```python
from build123d import *

# Parameters (mm, degrees)
SKETCH2_W             = 90
SKETCH2_H             = 23
BOSS_EXTRUDE2_DEPTH   = 5
SKETCH4_W             = 90
SKETCH4_H             = 5
BOSS_EXTRUDE3_DEPTH   = 35
M8X1_0_TAPPED_HOLE1_D = 7
M8X1_0_TAPPED_HOLE2_D = 7


with BuildPart() as part:
    # Sketch2 → Boss-Extrude2 (new body)
    with BuildSketch(Plane.XY):
        with Locations((0, -11.5)):
            Rectangle(SKETCH2_W, SKETCH2_H)
    extrude(amount=BOSS_EXTRUDE2_DEPTH)

    # Sketch4 → Boss-Extrude3 (add)
    with BuildSketch(Plane.XY.offset(5)):
        with Locations((0, -20.5)):
            Rectangle(SKETCH4_W, SKETCH4_H)
    extrude(amount=BOSS_EXTRUDE3_DEPTH)

    # M8x1.0 Tapped Hole1 (through all)
    with Locations(Plane.XY.offset(5)):
        with Locations((-25, -8), (25, -8)):
            Hole(M8X1_0_TAPPED_HOLE1_D / 2)

    # M8x1.0 Tapped Hole2 (through all)
    with Locations(Plane(origin=(0, -18, 0), x_dir=(1, 0, 0), z_dir=(0, 1, 0))):
        with Locations((-25, -25), (25, -25)):
            Hole(M8X1_0_TAPPED_HOLE2_D / 2)


solid = part.part
```
Source: CAD feature listing. Evaluate the final solid. Frame: model axes, mm. A direction names the side the tool comes from. Coordinates: 2 decimals unless noted, no trailing zeros. Write each loop counter-clockwise with the first axis right and the second up, starting at its lowest first coordinate (ties: lowest second). Pieces come first, ordered by that corner, then holes. Notation, with made-up numbers: (56, 54) - (66, 54) arc R6 cw to (66, 60) - close; hole circle Ø8 at (-16, 50). An arc over 180 degrees is marked (long way). Answer as a JSON object with one key per item and string values.
Q1. First-contact query: pin 1 Ø2 at (x, y) = (16.5, -9.5) entering from -Z; pin 2 Ø9 at (x, y) = (-9, -5.5) entering from +Z; pin 3 Ø10.5 at (x, z) = (-12.5, 27) entering from +Y. Flat tips, straight axial feed; report the tip coordinate or a pass-through.
Ans:
{"pin 1": "stops at z = 0", "pin 2": "stops at z = 5", "pin 3": "stops at y = -18"}
Q2. Material intervals for line 1 (X direction, y = -21.5, z = 25); line 2 (Y direction, x = -25, z = 3); line 3 (Z direction, x = -25, y = -20.75), sorted ascending. Write a range as [from, to].
Ans:
{"line 1": "x = [-45, -28.5], [-21.5, 21.5], [28.5, 45]", "line 2": "y = [-23, -11.5], [-4.5, 0]", "line 3": "z = [0, 21.5], [28.5, 40]"}
Q3. Section query D-D, the plane z = 20. Output: boundary loops of the cut face in (x, y).
Ans:
{"outline": "(-45, -23) - (45, -23) - (45, -18) - (-45, -18) - close"}
Q4. Section query B-B, the plane z = 25. Output: boundary loops of the cut face in (x, y).
Ans:
{"outline": "(-45, -23) - (-28.5, -23) - (-28.5, -18) - (-45, -18) - close; (-21.5, -23) - (21.5, -23) - (21.5, -18) - (-21.5, -18) - close; (28.5, -23) - (45, -23) - (45, -18) - (28.5, -18) - close"}
Q5. Draft query along Z for faces 1 (the flat face through (-1, -18, 22)), 2 (the flat face through (-1, -11, 0)), 3 (the cylindrical face through (23.12, -20.53, 22.05)). Return one class per face: released by +Z, released by -Z, zero draft, split by the parting line, or undercut.
Ans:
{"face 1": "zero draft", "face 2": "released by -Z", "face 3": "undercut"}
Q6. Set-up query: faces 4 (the flat face through (-1, -23, 20)), 5 (the flat face through (-1, -9, 5)). Return all of +Z, -Z, +X, -X, +Y, -Y with unobstructed straight access to the full face (end or side cutting, diameter ignored); none if empty.
Ans:
{"face 4": "+Z, -Z, +X, -X, -Y", "face 5": "+Z, +X, -X, +Y"}
Q7. Section query C-C, the plane y = -8. Output: boundary loops of the cut face in (x, z), plus the area to 3 significant figures.
Ans:
{"outline": "(-45, 0) - (-28.5, 0) - (-28.5, 5) - (-45, 5) - close; (-21.5, 0) - (21.5, 0) - (21.5, 5) - (-21.5, 5) - close; (28.5, 0) - (45, 0) - (45, 5) - (28.5, 5) - close", "area": "380 mm2"}
Q8. Section query A-A, the plane x = -25. Output: boundary loops of the cut face in (y, z), plus the area to 3 significant figures.
Ans:
{"outline": "(-23, 0) - (-11.5, 0) - (-11.5, 5) - (-18, 5) - (-18, 21.5) - (-23, 21.5) - close; (-23, 28.5) - (-18, 28.5) - (-18, 40) - (-23, 40) - close; (-4.5, 0) - (0, 0) - (0, 5) - (-4.5, 5) - close", "area": "220 mm2"}
